Geometry check sheet. Reference: the model listing, model coordinates, mm. Round coordinates to 2 decimals unless told otherwise and drop trailing zeros. Write each loop counter-clockwise with the first axis right and the second up, starting at its lowest first coordinate (ties: lowest second). Pieces come first, ordered by that corner, then holes.
Item 1: Cross-section at A-A (y = 35). Enter the section's corners in (x, z).
Item 2: Cross-section at B-B (x = 0). Enter the section's corners in (y, z).
Item 3: Depth check by flat-ended pin: P1, Ø2, axis at x = -11.5, y = 76.5, coming from the +Z side. Enter the tip coordinate at first touch or a pass-through.
Item 4: Scan lines: probe 1 along Z at (x, y) = (0, 9); probe 2 along X at (y, z) = (79.5, -1); probe 3 along X at (y, z) = (29, -4.25). Record each from-to range of solid material in increasing order.
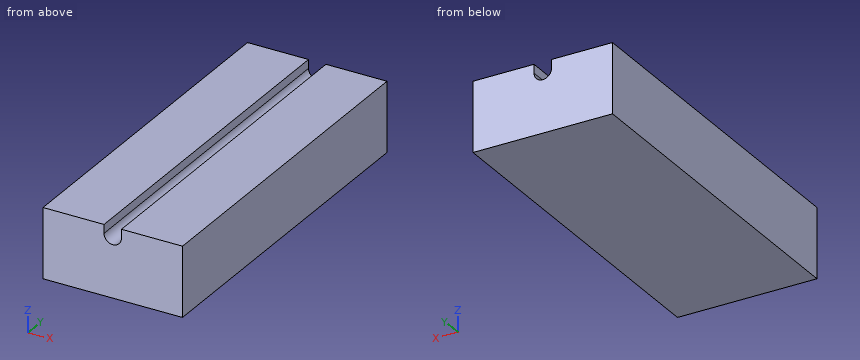
from build123d import *

# Parameters (mm, degrees)
F0_W     = 40
F0_H     = 100
F1_DEPTH = 20
F3_DEPTH = 100


with BuildPart() as f1:
    # F0 (on Top) → F1 (new body)
    with BuildSketch(Plane.XY):
        with Locations((0, 40.365882)):
            Rectangle(F0_W, F0_H)
    extrude(amount=-F1_DEPTH)

    # F2 (on face) → F3 (cut, through all)
    with BuildSketch(Plane.XZ.offset(9.634118)):
        with BuildLine():
            ThreePointArc((-2.5, -2.5), (0, -5), (2.5, -2.5))
            ThreePointArc((2.5, -2.5), (0, 0), (-2.5, -2.5))
        make_face()
        with BuildLine():
            ThreePointArc((0, 0), (1.767767, -0.732233), (2.5, -2.5))
            Line((2.5, -2.5), (2.5, 0))
            Line((2.5, 0), (0, 0))
        make_face()
        with BuildLine():
            Line((-2.5, 0), (-2.5, -2.5))
            ThreePointArc((-2.5, -2.5), (-1.767767, -0.732233), (0, 0))
            Line((0, 0), (-2.5, 0))
        make_face()
    extrude(amount=-F3_DEPTH, mode=Mode.SUBTRACT)


solid = f1.part
Resolved:
1. outline: (-20, -20) - (20, -20) - (20, 0) - (2.5, 0) - (2.5, -2.5) arc R2.5 cw to (-2.5, -2.5) - (-2.5, 0) - (-20, 0) - close
2. outline: (-9.63, -20) - (90.37, -20) - (90.37, -5) - (-9.63, -5) - close
3. P1: stops at z = 0
4. probe 1: z = -20 to -5
4. probe 2: x = -20 to -2.5, 2.5 to 20
4. probe 3: x = -20 to -1.79, 1.79 to 20
